Could you check a few things on this model? Use its own coordinates, in mm. Face numbers are marked on the shaded views. A direction names the side the tool comes from. Round coordinates to 2 decimals unless told otherwise and drop trailing zeros. Order: outer loops, then holes, each group sorted by start corner. A loop starts at its lowest first (then second) coordinate and runs counter-clockwise, first axis right, second up. Notation, with made-up numbers: (43.5, 55) -> (77.5, 55) arc R27 ccw to (77.5, 81) -> close; hole circle Ø7 at (-14, 87). An arc over 180 degrees is marked (long way). One line per question, with ' | ' between items.
```python
from build123d import *

# Parameters (mm, degrees)
ESQUISSE1_R             = 15
BOSS_EXTRU_1_DEPTH      = 20
ESQUISSE2_R             = 10
ENL_V_MAT_EXTRU_1_DEPTH = 12
ESQUISSE3_R             = 3
ENL_V_MAT_EXTRU_2_DEPTH = 12
ESQUISSE4_R             = 1.5
ENL_V_MAT_EXTRU_3_DEPTH = 8


with BuildPart() as part:
    # Esquisse1 → Boss.-Extru.1 (new body)
    with BuildSketch(Plane(origin=(0, 0, 0), x_dir=(1, 0, 0), z_dir=(0, 1, 0))):
        with Locations(Location((0, 0, 0), (0, 0, 270))):
            Circle(ESQUISSE1_R)
    extrude(amount=BOSS_EXTRU_1_DEPTH)

    # Esquisse2 → Enlèv. mat.-Extru.1 (cut)
    with BuildSketch(Plane(origin=(0, 0, 0), x_dir=(-1, 0, 0), z_dir=(0, -1, 0))):
        with Locations(Location((0, 0, 0), (0, 0, 90))):
            Circle(ESQUISSE2_R)
    extrude(amount=-ENL_V_MAT_EXTRU_1_DEPTH, mode=Mode.SUBTRACT)

    # Esquisse3 → Enlèv. mat.-Extru.2 (cut)
    with BuildSketch(Plane(origin=(0, 12, 0), x_dir=(-1, 0, 0), z_dir=(0, -1, 0))):
        with Locations(Location((0, 0, 0), (0, 0, 90))):
            Circle(ESQUISSE3_R)
    extrude(amount=-ENL_V_MAT_EXTRU_2_DEPTH, mode=Mode.SUBTRACT)

    # Esquisse4 → Enlèv. mat.-Extru.3 (cut)
    with BuildSketch(Plane(origin=(0, 0, 0), x_dir=(-1, 0, 0), z_dir=(0, -1, 0))):
        with Locations(Location((-12.7, 0, 0), (0, 0, 90))):
            Circle(ESQUISSE4_R)
        with Locations(Location((0, -12.7, 0), (0, 0, 90))):
            Circle(ESQUISSE4_R)
        with Locations(Location((12.7, 0, 0), (0, 0, 90))):
            Circle(ESQUISSE4_R)
        with Locations(Location((0, 12.7, 0), (0, 0, 90))):
            Circle(ESQUISSE4_R)
    extrude(amount=-ENL_V_MAT_EXTRU_3_DEPTH, mode=Mode.SUBTRACT)


solid = part.part
```
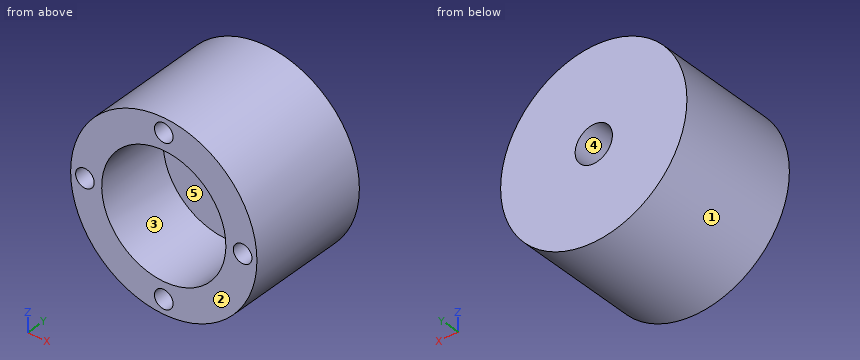
1. I want a section at C-C on z = 12.7. List the corners of the cut face in (x, y) for me, and give its area (3 significant figures).
From the geometry:
outline: (-7.98, 0) -> (-1.5, 0) -> (-1.5, 8) -> (1.5, 8) -> (1.5, 0) -> (7.98, 0) -> (7.98, 20) -> (-7.98, 20) -> close | area: 295 mm²
2. I'm going to push flat-ended pins straight in: pin 1 (2 mm diameter, centred on y = 9, z = 9, fed in from +X); pin 2 (4 mm diameter, centred on y = 12, z = -3.5, fed in from -X); pin 3 (12 mm diameter, centred on x = -6.5, y = 16.5, fed in from +Z). Where does each tip first touch, or does it pass through?
From the geometry:
pin 1: stops at x = 12.69 | pin 2: stops at x = -14.92 | pin 3: stops at z = 14.99
3. I want a section at D-D on y = 7.5. List the corners of the cut face in (x, z) for me, and give its area (3 significant figures).
From the geometry:
outline: circle Ø30 at (0, 0); hole circle Ø3 at (-12.7, 0); hole circle Ø20 at (0, 0); hole circle Ø3 at (0, -12.7); hole circle Ø3 at (0, 12.7); hole circle Ø3 at (12.7, 0) | area: 364 mm²
4. I need wall thicknesses on probe 1 along X at (y, z) = (3.25, 0); probe 2 along X at (y, z) = (12.75, 0); probe 3 along Y at (x, z) = (-5, 2.75). Which ranges of each line are inside material? Lowest first, please.
From the geometry:
probe 1: x = -15 to -14.2, -11.2 to -10, 10 to 11.2, 14.2 to 15 | probe 2: x = -15 to -3, 3 to 15 | probe 3: y = 12 to 20
5. On a 3-axis mill with a long thin cutter (end or side, diameter ignored), from which of +Z, -Z, +X, -X, +Y, -Y can I reach the whole of each face in a straight line? I mean the marked faces 4 and 5. Say none if no direction works.
From the geometry:
face 4: +Y, -Y | face 5: -Y
6. If we mould it in two halves opening along X, with no side actions, what happens to the marked faces 1, 2 and 3? For each: pulls with the +X half, pulls with the -X half, needs draft (parallel to the pull), parting line crosses it, or undercut.
From the geometry:
face 1: parting line crosses it | face 2: needs draft | face 3: undercut
7. I want a section at B-B on y = 16. List the corners of the cut face in (x, z) for me, and give its area (3 significant figures).
From the geometry:
outline: circle Ø30 at (0, 0); hole circle Ø6 at (0, 0) | area: 679 mm²
8. I want a section at A-A on x = 0. List the corners of the cut face in (y, z) for me.
From the geometry:
outline: (0, -15) -> (20, -15) -> (20, -3) -> (12, -3) -> (12, -10) -> (0, -10) -> (0, -11.2) -> (8, -11.2) -> (8, -14.2) -> (0, -14.2) -> close; (0, 10) -> (12, 10) -> (12, 3) -> (20, 3) -> (20, 15) -> (0, 15) -> (0, 14.2) -> (8, 14.2) -> (8, 11.2) -> (0, 11.2) -> close
